from build123d import *

# Parameters (mm, degrees)
BOSS_EXTRU_1_DEPTH      = 20
BOSS_EXTRU_2_DEPTH      = 2
ESQUISSE3_R             = 6.5
BOSS_EXTRU_3_DEPTH      = 1
ESQUISSE4_R             = 5.5
BOSS_EXTRU_4_DEPTH      = 0.25
ESQUISSE5_R             = 3
BOSS_EXTRU_5_DEPTH      = 4
ENL_V_START             = -4
ENL_V_MAT_EXTRU_1_DEPTH = 4
ENL_V_MAT_EXTRU_2_DEPTH = 46.716517803
CONG_1_R                = 1.5
CHANFREIN1_SIZE         = 2
CONG_2_R                = 0.5


with BuildPart() as part:
    # Esquisse1 → Boss.-Extru.1 (new body)
    with BuildSketch(Plane(origin=(0, 0, 0), x_dir=(0, 0, -1), z_dir=(1, 0, 0))):
        Polygon((0, -20), (0, 20), (28, 20), (28, 27), (31, 27), (31, 20), (37, 20), (37, -20), (31, -20), (31, -27), (28, -27), (28, -20), align=None)
    extrude(amount=BOSS_EXTRU_1_DEPTH)

    # Esquisse2 → Boss.-Extru.2 (add)
    with BuildSketch(Plane(origin=(0, 0, -37), x_dir=(-1, 0, 0), z_dir=(0, 0, -1))):
        with BuildLine():
            ThreePointArc((-0.5, 6.877501001), (-10, 20), (-19.5, 6.877501001))
            Line((-19.5, 6.877501001), (-19.5, -15))
            Line((-19.5, -15), (-14.898979486, -15))
            ThreePointArc((-14.898979486, -15), (-10, -17), (-5.101020514, -15))
            Line((-5.101020514, -15), (-0.5, -15))
            Line((-0.5, -15), (-0.5, 6.877501001))
        make_face()
    extrude(amount=BOSS_EXTRU_2_DEPTH)

    # Esquisse3 → Boss.-Extru.3 (add)
    with BuildSketch(Plane(origin=(0, 0, -39), x_dir=(-1, 0, 0), z_dir=(0, 0, -1))):
        with Locations((-10, 10)):
            Circle(ESQUISSE3_R)
    extrude(amount=BOSS_EXTRU_3_DEPTH)

    # Esquisse4 → Boss.-Extru.4 (add)
    with BuildSketch(Plane(origin=(0, 0, -40), x_dir=(-1, 0, 0), z_dir=(0, 0, -1))):
        with Locations((-10, 10)):
            Circle(ESQUISSE4_R)
    extrude(amount=BOSS_EXTRU_4_DEPTH)

    # Esquisse5 → Boss.-Extru.5 (add)
    with BuildSketch(Plane(origin=(0, 0, -40.25), x_dir=(-1, 0, 0), z_dir=(0, 0, -1))):
        with Locations((-10, 10)):
            Circle(ESQUISSE5_R)
    extrude(amount=BOSS_EXTRU_5_DEPTH)

    # Esquisse6 → Enlèv. mat.-Extru.1 (cut)
    with BuildSketch(Plane(origin=(0, 0, -44.25), x_dir=(-1, 0, 0), z_dir=(0, 0, -1)).offset(ENL_V_START)):
        with BuildLine():
            ThreePointArc((-8.97393957, 12.819077862), (-9.479055467, 12.954423259), (-10, 13))
            Line((-10, 13), (-9.565879556, 12.462019383))
            Line((-9.565879556, 12.462019383), (-8.97393957, 12.819077862))
        make_face()
        with BuildLine():
            Line((-10.434120444, 12.462019383), (-10, 13))
            ThreePointArc((-10, 13), (-10.520944533, 12.954423259), (-11.02606043, 12.819077862))
            Line((-11.02606043, 12.819077862), (-10.434120444, 12.462019383))
        make_face()
        with BuildLine():
            ThreePointArc((-8.071637171, 12.298133329), (-8.5, 12.598076211), (-8.97393957, 12.819077862))
            Line((-8.97393957, 12.819077862), (-8.75, 12.165063509))
            Line((-8.75, 12.165063509), (-8.071637171, 12.298133329))
        make_face()
        with BuildLine():
            Line((-11.25, 12.165063509), (-11.02606043, 12.819077862))
            ThreePointArc((-11.02606043, 12.819077862), (-11.5, 12.598076211), (-11.928362829, 12.298133329))
            Line((-11.928362829, 12.298133329), (-11.25, 12.165063509))
        make_face()
        with BuildLine():
            ThreePointArc((-7.401923789, 11.5), (-7.701866671, 11.928362829), (-8.071637171, 12.298133329))
            Line((-8.071637171, 12.298133329), (-8.084888892, 11.606969024))
            Line((-8.084888892, 11.606969024), (-7.401923789, 11.5))
        make_face()
        with BuildLine():
            Line((-11.915111108, 11.606969024), (-11.928362829, 12.298133329))
            ThreePointArc((-11.928362829, 12.298133329), (-12.298133329, 11.928362829), (-12.598076211, 11.5))
            Line((-12.598076211, 11.5), (-11.915111108, 11.606969024))
        make_face()
        with BuildLine():
            ThreePointArc((-7.045576741, 10.520944533), (-7.180922138, 11.02606043), (-7.401923789, 11.5))
            Line((-7.401923789, 11.5), (-7.650768448, 10.855050358))
            Line((-7.650768448, 10.855050358), (-7.045576741, 10.520944533))
        make_face()
        with BuildLine():
            Line((-12.349231552, 10.855050358), (-12.598076211, 11.5))
            ThreePointArc((-12.598076211, 11.5), (-12.819077862, 11.02606043), (-12.954423259, 10.520944533))
            Line((-12.954423259, 10.520944533), (-12.349231552, 10.855050358))
        make_face()
        with BuildLine():
            ThreePointArc((-7.045576741, 9.479055467), (-7, 10), (-7.045576741, 10.520944533))
            Line((-7.045576741, 10.520944533), (-7.5, 10))
            Line((-7.5, 10), (-7.045576741, 9.479055467))
        make_face()
        with BuildLine():
            Line((-12.5, 10), (-12.954423259, 10.520944533))
            ThreePointArc((-12.954423259, 10.520944533), (-13, 10), (-12.954423259, 9.479055467))
            Line((-12.954423259, 9.479055467), (-12.5, 10))
        make_face()
        with BuildLine():
            Line((-12.349231552, 9.144949642), (-12.954423259, 9.479055467))
            ThreePointArc((-12.954423259, 9.479055467), (-12.819077862, 8.97393957), (-12.598076211, 8.5))
            Line((-12.598076211, 8.5), (-12.349231552, 9.144949642))
        make_face()
        with BuildLine():
            ThreePointArc((-7.401923789, 8.5), (-7.180922138, 8.97393957), (-7.045576741, 9.479055467))
            Line((-7.045576741, 9.479055467), (-7.650768448, 9.144949642))
            Line((-7.650768448, 9.144949642), (-7.401923789, 8.5))
        make_face()
        with BuildLine():
            Line((-11.915111108, 8.393030976), (-12.598076211, 8.5))
            ThreePointArc((-12.598076211, 8.5), (-12.298133329, 8.071637171), (-11.928362829, 7.701866671))
            Line((-11.928362829, 7.701866671), (-11.915111108, 8.393030976))
        make_face()
        with BuildLine():
            ThreePointArc((-8.071637171, 7.701866671), (-7.701866671, 8.071637171), (-7.401923789, 8.5))
            Line((-7.401923789, 8.5), (-8.084888892, 8.393030976))
            Line((-8.084888892, 8.393030976), (-8.071637171, 7.701866671))
        make_face()
        with BuildLine():
            Line((-11.25, 7.834936491), (-11.928362829, 7.701866671))
            ThreePointArc((-11.928362829, 7.701866671), (-11.5, 7.401923789), (-11.02606043, 7.180922138))
            Line((-11.02606043, 7.180922138), (-11.25, 7.834936491))
        make_face()
        with BuildLine():
            ThreePointArc((-8.97393957, 7.180922138), (-8.5, 7.401923789), (-8.071637171, 7.701866671))
            Line((-8.071637171, 7.701866671), (-8.75, 7.834936491))
            Line((-8.75, 7.834936491), (-8.97393957, 7.180922138))
        make_face()
        with BuildLine():
            Line((-10.434120444, 7.537980617), (-11.02606043, 7.180922138))
            ThreePointArc((-11.02606043, 7.180922138), (-10.520944533, 7.045576741), (-10, 7))
            Line((-10, 7), (-10.434120444, 7.537980617))
        make_face()
        with BuildLine():
            ThreePointArc((-10, 7), (-9.479055467, 7.045576741), (-8.97393957, 7.180922138))
            Line((-8.97393957, 7.180922138), (-9.565879556, 7.537980617))
            Line((-9.565879556, 7.537980617), (-10, 7))
        make_face()
    extrude(amount=ENL_V_MAT_EXTRU_1_DEPTH, mode=Mode.SUBTRACT)

    # Esquisse7 → Enlèv. mat.-Extru.2 (cut, through all)
    with BuildSketch(Plane(origin=(0, 0, -31), x_dir=(-1, 0, 0), z_dir=(0, 0, -1))):
        with BuildLine():
            Line((-4, 27), (-6, 27))
            Line((-6, 27), (-6, 26.291287847))
            ThreePointArc((-6, 26.291287847), (-5, 21.5), (-4, 26.291287847))
            Line((-4, 26.291287847), (-4, 27))
        make_face()
        with BuildLine():
            Line((-14, 26.291287847), (-14, 27))
            Line((-14, 27), (-16, 27))
            Line((-16, 27), (-16, 26.291287847))
            ThreePointArc((-16, 26.291287847), (-15, 21.5), (-14, 26.291287847))
        make_face()
        with BuildLine():
            Line((-6, -27), (-4, -27))
            Line((-4, -27), (-4, -26.291287847))
            ThreePointArc((-4, -26.291287847), (-5, -21.5), (-6, -26.291287847))
            Line((-6, -26.291287847), (-6, -27))
        make_face()
        with BuildLine():
            Line((-16, -27), (-14, -27))
            Line((-14, -27), (-14, -26.291287847))
            ThreePointArc((-14, -26.291287847), (-15, -21.5), (-16, -26.291287847))
            Line((-16, -26.291287847), (-16, -27))
        make_face()
    extrude(amount=-ENL_V_MAT_EXTRU_2_DEPTH, mode=Mode.SUBTRACT)

    # Congé1
    cong_1_edges = [part.edges().sort_by_distance(p)[0] for p in [
        (0, -27, -29.5),
        (0, 27, -29.5),
        (20, 27, -29.5),
        (20, -27, -29.5),
    ]]
    fillet(cong_1_edges, radius=CONG_1_R)

    # Chanfrein1
    chanfrein1_edges = [part.edges().sort_by_distance(p)[0] for p in [
        (0, 0, 0),
        (10, -20, 0),
        (10, 20, 0),
        (20, 0, 0),
    ]]
    chamfer(chanfrein1_edges, length=CHANFREIN1_SIZE)

    # Congé2
    cong_2_edges = [part.edges().sort_by_distance(p)[0] for p in [
        (20, 20, -34),
        (0, 20, -15),
        (0, 20, -34),
        (0, -20, -34),
        (20, 20, -15),
        (20, -20, -15),
        (0, -20, -15),
        (20, -20, -34),
    ]]
    fillet(cong_2_edges, radius=CONG_2_R)


solid = part.part
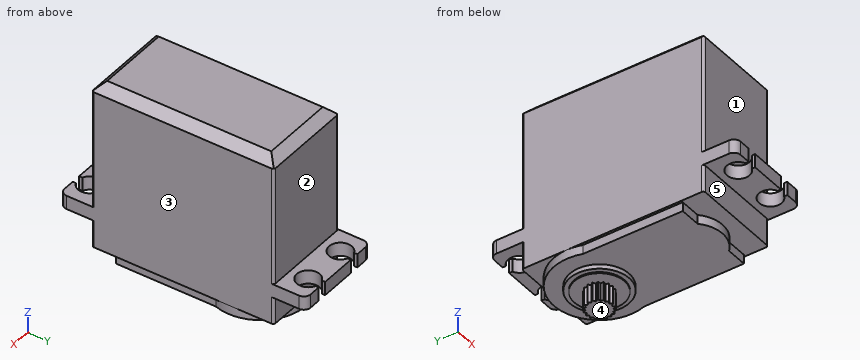
Can you work these out from the model? Positions are in its coordinate system, mm. Face numbers are marked on the shaded views. A direction names the side the tool comes from. Coordinates: 2 decimals unless noted, no trailing zeros. Write each loop counter-clockwise with the first axis right and the second up, starting at its lowest first coordinate (ties: lowest second). Pieces come first, ordered by that corner, then holes. Notation, with made-up numbers: (33.5, 26.5) -> (65.5, 26.5) arc R17 ccw to (65.5, 46.5) -> close; hole circle Ø10 at (81, 77). An arc over 180 degrees is marked (long way). Answer as CSV lines item,"result".
1) If we section it at A-A on y = 24: Please give me the cut outline in (x, z).
Check result:
outline,"(0, -31) -> (2.5, -31) -> (2.5, -28) -> (0, -28) -> close; (7.5, -31) -> (12.5, -31) -> (12.5, -28) -> (7.5, -28) -> close; (17.5, -31) -> (20, -31) -> (20, -28) -> (17.5, -28) -> close"
2) Will these pins go through, and if not, where does the flat tip stop? P1, Ø1.6, axis at y = -4.5, z = -38, coming from the -X side; P2, Ø1.8, axis at x = 9, z = -35.5, coming from the -Y side; P3, Ø11, axis at x = 6.5, y = 12.5, coming from the -Z side; P4, Ø0.6, axis at y = 26.5, z = -29.5, coming from the -X side.
Check result:
P1,"x = 0.5"
P2,"y = -20"
P3,"z = -44.25"
P4,"x = 0.17"
3) If I drill on line 1 (X direction, y = -24, z = -29.9); line 2 (Y direction, x = 15.75, z = -3.5); line 3 (Z direction, x = 15.25, y = 11), over which ranges is the centre line in solid material (lowest first)? Write a range as from..to.
Check result:
line 1,"0..2.5, 7.5..12.5, 17.5..20"
line 2,"-20..20"
line 3,"-40.25..0"
4) On a 3-axis mill with a long thin cutter (end or side, diameter ignored), from which of +Z, -Z, +X, -X, +Y, -Y can I reach the whole of each face in a straight line? I mean the marked faces 1, 2, 3, 4 and 5. Say none if no direction works.
Check result:
face 1,"+Z, +X, -X, -Y"
face 2,"+Z, +X, -X, +Y"
face 3,"+Z, -Z, +X, +Y, -Y"
face 4,"-Z, +X, -X, +Y, -Y"
face 5,"-Z, +X, -X, -Y"
5) If we section it at C-C on y = -7: Please give me the cut outline in (x, z), then the cut area to 3 significant figures.
Check result:
outline,"(0, -37) -> (0.5, -37) -> (0.5, -39) -> (19.5, -39) -> (19.5, -37) -> (20, -37) -> (20, -2) -> (18, 0) -> (2, 0) -> (0, -2) -> close"
area,"774 mm²"
6) If we section it at B-B on z = -24.5: Please give me the cut outline in (x, y), then the cut area to 3 significant figures.
Check result:
outline,"(0, -19.5) arc R0.5 ccw to (0.5, -20) -> (19.5, -20) arc R0.5 ccw to (20, -19.5) -> (20, 19.5) arc R0.5 ccw to (19.5, 20) -> (0.5, 20) arc R0.5 ccw to (0, 19.5) -> close"
area,"800 mm²"
